Source: CAD feature listing. Evaluate the final solid. Frame: model axes, mm. A direction names the side the tool comes from. Round coordinates to 2 decimals unless told otherwise and drop trailing zeros. Write each loop counter-clockwise with the first axis right and the second up, starting at its lowest first coordinate (ties: lowest second). Pieces come first, ordered by that corner, then holes. Notation, with made-up numbers: (41, -5.5) -> (67, -5.5) arc R24 cw to (67, 9.5) -> close; hole circle Ø10 at (43.5, 68). An arc over 180 degrees is marked (long way). Put each result on its own line as item: value.
```python
from build123d import *

# Parameters (mm, degrees)
SKETCH072_R     = 2.7
PAD031_DEPTH    = 10
SKETCH069_R     = 2.6
POCKET028_DEPTH = 8
SKETCH070_R     = 3
POCKET029_DEPTH = 1
SKETCH073_R     = 2
POCKET030_DEPTH = 8


with BuildPart() as loft004:
    # Sketch072 → Loft004 section 0
    with BuildSketch(Plane.XY.offset(18)):
        with Locations((-5, 0)):
            Circle(SKETCH072_R)
    # Sketch071 → Loft004 section 1
    with BuildSketch(Plane.XY.offset(38)):
        with BuildLine():
            ThreePointArc((-6.3, 3), (-9.3, 0), (-6.3, -3))
            Line((-6.3, -3), (-3.3, -3))
            ThreePointArc((-3.3, -3), (-0.3, 0), (-3.3, 3))
            Line((-3.3, 3), (-6.3, 3))
        make_face()
    loft()


with BuildPart() as part_mirroring004:
    # Part__Mirroring004: instance of Loft004
    add(loft004.part.mirror(Plane(origin=(0, 0, 0), x_dir=(0, -1, 0), z_dir=(1, 0, 0))))


with BuildPart() as fusion004:
    # Fusion004 base: copy of Loft004
    add(loft004.part)

    # Fusion004: union Part__Mirroring004
    add(part_mirroring004.part)


with BuildPart() as cut003:
    # Sketch068 → Pad031 (new body)
    with BuildSketch(Plane.XZ):
        Polygon((-16, 4), (-9.85, 4), (-9.85, 7), (-9.85, 8.6), (-9, 8.6), (-9, 10.6), (9, 10.6), (9, 8.6), (9.85, 8.6), (9.85, 7), (9.85, 4), (16, 4), (16, 12), (12.15, 15.85), (12.15, 26.306086), (16.15, 30), (16.15, 38), (-16.15, 38), (-16.15, 30), (-12.15, 26.306086), (-12.15, 15.85), (-16, 12), align=None)
    extrude(amount=PAD031_DEPTH)

    # Sketch069 (on Face7 of Pad031) → Pocket028 (cut)
    with BuildSketch(Plane(origin=(0, 0, 10.6), x_dir=(1, 0, 0), z_dir=(0, 0, -1))):
        with Locations((-5, 5)):
            Circle(SKETCH069_R)
        with Locations((5, 5)):
            Circle(SKETCH069_R)
    extrude(amount=-POCKET028_DEPTH, mode=Mode.SUBTRACT)

    # Sketch070 (on Face11 of Pocket028) → Pocket029 (cut)
    with BuildSketch(Plane(origin=(0, 0, 10.6), x_dir=(1, 0, 0), z_dir=(0, 0, -1))):
        with Locations((-5, 5)):
            Circle(SKETCH070_R)
        with Locations((5, 5)):
            Circle(SKETCH070_R)
    extrude(amount=-POCKET029_DEPTH, mode=Mode.SUBTRACT)

    # Sketch073 (on Face22 of Pocket029) → Pocket030 (cut)
    with BuildSketch(Plane(origin=(0, 0, 38), x_dir=(-1, 0, 0), z_dir=(0, 0, 1))):
        with Locations((-12, 5)):
            Circle(SKETCH073_R)
        with Locations((12, 5)):
            Circle(SKETCH073_R)
    extrude(amount=-POCKET030_DEPTH, mode=Mode.SUBTRACT)


with BuildPart() as cut003_1:
    # Body025 placement: moved
    add(cut003.part.moved(Location((0, 5, 0))))

    # Cut003: cut Fusion004
    add(fusion004.part, mode=Mode.SUBTRACT)


with BuildPart() as cut003_2:
    # Cut003 placement: moved
    add(cut003_1.part.moved(Location((0, -184.33, 0))))


solid = cut003_2.part
```
Q1. Cut plane A-A on y = -180.75. Output: boundary loops of the cut face in (x, z), and give its area (3 significant figures).
Ans:
outline: (-16.15, 30) -> (-12.15, 26.31) -> (-12.15, 15.85) -> (-16, 12) -> (-16, 4) -> (-9.85, 4) -> (-9.85, 8.6) -> (-9, 8.6) -> (-9, 10.6) -> (9, 10.6) -> (9, 8.6) -> (9.85, 8.6) -> (9.85, 4) -> (16, 4) -> (16, 12) -> (12.15, 15.85) -> (12.15, 26.31) -> (16.15, 30) -> (16.15, 38) -> (-16.15, 38) -> close
area: 855 mm^2
Q2. Reachability of faces 5 (the cylindrical face through (4.609, -187.304, 11.093)), 6 (the flat face through (14, -184, 14)), 7 (the flat face through (-16, -184, 8)) from +Z, -Z, +X, -X, +Y, -Y: full face, straight path, thin tool, end or side. Return the list, or none.
Ans:
face 5: -Z
face 6: +X, +Y, -Y
face 7: -Z, -X, +Y, -Y
Q3. Pin query (flat end, axial travel): pin 1 (5 mm diameter, centred on y = -184.5, z = 21.5, fed in from +X); pin 2 (1.4 mm diameter, centred on y = -183, z = 7, fed in from +X); pin 3 (2.5 mm diameter, centred on y = -184.5, z = 7, fed in from -X); pin 4 (4 mm diameter, centred on y = -186, z = 29, fed in from -X). Return the tip coordinate at first contact, or that it passes through.
Ans:
pin 1: stops at x = 12.15
pin 2: stops at x = 16
pin 3: stops at x = -16
pin 4: stops at x = -16.15
Q4. Cut plane C-C on y = -183. Give the number of separate pieces and of enclosed holes in the cut face, and give its area (3 significant figures).
Ans:
separate pieces: 3
enclosed holes: 0
area: 478 mm^2
Q5. Material intervals for line 1 (X direction, y = -184.33, z = 10.8); line 2 (X direction, y = -184.33, z = 16); line 3 (Y direction, x = 5, z = 16), sorted ascending. Write a range as [from, to].
Ans:
line 1: x = [-16, -8], [-2, 2], [8, 16]
line 2: x = [-12.15, -7.6], [-2.4, 2.4], [7.6, 12.15]
line 3: y = [-189.33, -186.93], [-181.73, -179.33]
Q6. Cut plane B-B on x = -13. Output: boundary loops of the cut face in (y, z), and give its area (3 significant figures).
Ans:
outline: (-189.33, 4) -> (-179.33, 4) -> (-179.33, 15) -> (-189.33, 15) -> close; (-189.33, 27.09) -> (-179.33, 27.09) -> (-179.33, 38) -> (-182.6, 38) -> (-182.6, 30) -> (-186.06, 30) -> (-186.06, 38) -> (-189.33, 38) -> close
area: 191 mm^2
Q7. Draft query along Z for faces 1 (the flat face through (-9.4, -184.3, 8.6)), 2 (the flat face through (-14.2, -184.3, 28.2)), 3 (the flat face through (-12.15, -184, 21)), 4 (the flat face through (-16.15, -184, 34)). Return one class per face: +Z half, -Z half, draft (parallel to the pull), parting line (faces both ways), or undercut.
Ans:
face 1: -Z half
face 2: undercut
face 3: undercut
face 4: draft
